Input: part model. Units: mm. Frame: model coordinates. Round coordinates to 2 decimals unless told otherwise and drop trailing zeros. Write each loop counter-clockwise with the first axis right and the second up, starting at its lowest first coordinate (ties: lowest second). Pieces come first, ordered by that corner, then holes. Notation, with made-up numbers: (-5, 84) -> (3, 84) arc R27 cw to (3, 105) -> close; hole circle Ø2 at (-26, -28). An arc over 180 degrees is marked (long way). Use CSV: the item, a comma, the result in double quotes.
```python
from build123d import *

# Parameters (mm, degrees)
BOSS_EXTRUDE1_DEPTH = 40


with BuildPart() as part:
    # Sketch1 → Boss-Extrude1 (new body, symmetric)
    with BuildSketch(Plane.XY):
        Polygon((576.530281573, 118.813515451), (-381.24605126, 118.813515451), (-614.016581357, -25.106107257), (-614.016581357, -77.668223147), (-386.909457622, -118.813515451), (-159.802333887, -118.813515451), (-45.574406616, -5.335493482), (524.577232755, 38.483934534), (614.016581357, 38.369843561), (614.016581357, 118.813515451), align=None)
    extrude(amount=BOSS_EXTRUDE1_DEPTH, both=True)


solid = part.part
```
Item 1: Section query A-A on z = 26. Return the cut outline in (x, y), plus the area to 3 significant figures.
Worked answers:
outline,"(-614.02, -77.67) -> (-386.91, -118.81) -> (-159.8, -118.81) -> (-45.57, -5.34) -> (524.58, 38.48) -> (614.02, 38.37) -> (614.02, 118.81) -> (-381.25, 118.81) -> (-614.02, -25.11) -> close"
area,"173,000 mm²"
Item 2: Line query: line 1 (Y direction, x = -45, z = 20); line 2 (Y direction, x = 119, z = 26); line 3 (X direction, y = 55, z = -27). Output: solid intervals per line, ascending.
Worked answers:
line 1,"y = -5.29 to 118.81"
line 2,"y = 7.31 to 118.81"
line 3,"x = -484.46 to 614.02"
Item 3: First-contact query: pin 1 Ø5 at (y, z) = (-67.5, -10) entering from +X; pin 2 Ø1.5 at (y, z) = (-9, -12) entering from -X. Flat tips, straight axial feed; report the tip coordinate or a pass-through.
Worked answers:
pin 1,"stops at x = -105.63"
pin 2,"stops at x = -589.18"
Item 4: Section query B-B on y = 79. Return the cut outline in (x, z), plus the area to 3 significant figures.
Worked answers:
outline,"(-445.64, -40) -> (614.02, -40) -> (614.02, 40) -> (-445.64, 40) -> close"
area,"84,800 mm²"
Item 5: Section query C-C on x = 231.5. Return the cut outline in (y, z).
Worked answers:
outline,"(15.96, -40) -> (118.81, -40) -> (118.81, 40) -> (15.96, 40) -> close"
